```python
from build123d import *

# Parameters (mm, degrees)
SKETCH_1_R          = 15
EXTRUDE_1_DEPTH     = 6
SKETCH_2_R          = 1.6
CUT_EXTRUDE_1_DEPTH = 23.045407685
SKETCH_3_R          = 3.05
CUT_EXTRUDE_2_DEPTH = 1.2
SKETCH_4_R          = 4
EXTRUDE_2_DEPTH     = 25


with BuildPart() as part:
    # 草图1 → 凸台-拉伸1 (new body)
    with BuildSketch(Plane.XY):
        Circle(SKETCH_1_R)
    extrude(amount=EXTRUDE_1_DEPTH)

    # 草图2 → 切除-拉伸1 (cut, through all)
    with BuildSketch(Plane.XY.offset(6)):
        with Locations((0, 11.5)):
            Circle(SKETCH_2_R)
        with Locations((9.959292144, -5.75)):
            Circle(SKETCH_2_R)
        with Locations((-9.959292144, -5.75)):
            Circle(SKETCH_2_R)
        with Locations((-9.09326674, 5.25)):
            Circle(SKETCH_2_R)
        with Locations((9.09326674, 5.25)):
            Circle(SKETCH_2_R)
        with Locations((0, -10.5)):
            Circle(SKETCH_2_R)
    extrude(amount=-CUT_EXTRUDE_1_DEPTH, mode=Mode.SUBTRACT)

    # 草图3 → 切除-拉伸2 (cut)
    with BuildSketch(Plane.XY.offset(6)):
        with Locations((-9.09326674, 5.25)):
            Circle(SKETCH_3_R)
        with Locations((0, 11.5)):
            Circle(SKETCH_3_R)
        with Locations((9.09326674, 5.25)):
            Circle(SKETCH_3_R)
        with Locations((9.959292144, -5.75)):
            Circle(SKETCH_3_R)
        with Locations((0, -10.5)):
            Circle(SKETCH_3_R)
        with Locations((-9.959292144, -5.75)):
            Circle(SKETCH_3_R)
    extrude(amount=-CUT_EXTRUDE_2_DEPTH, mode=Mode.SUBTRACT)

    # 草图4 → 凸台-拉伸2 (add)
    with BuildSketch(Plane.XY.offset(6)):
        Circle(SKETCH_4_R)
    extrude(amount=EXTRUDE_2_DEPTH)

    # 草图5 → 旋转2 (revolve)
    with BuildSketch(Plane(origin=(0, 0, 0), x_dir=(1, 0, 0), z_dir=(0, 1, 0))):
        with BuildLine():
            Line((0, -29), (0, -45.9))
            ThreePointArc((0, -45.9), (-8.45, -37.45), (0, -29))
        make_face()
    revolve(axis=Axis((0, 0, 0), (0, 0, 1)))


solid = part.part
```
Input: part model. Units: mm. Frame: model coordinates. A direction names the side the tool comes from. Give positions to 0.01 mm unless a question says otherwise; leave off trailing zeros. Order: outer loops, then holes, each group sorted by start corner. A loop starts at its lowest first (then second) coordinate and runs counter-clockwise, first axis right, second up.
1. Material intervals for L1, parallel to Y at x = 0, z = 1.2; L2, parallel to Y at x = 0, z = 5.75; L3, parallel to Z at x = -5.75, y = 12.75, sorted ascending.
Derived:
L1: y = -15 to -12.1, -8.9 to 9.9, 13.1 to 15
L2: y = -15 to -13.55, -7.45 to 8.45, 14.55 to 15
L3: z = 0 to 6
2. Section B-B on y = 0. Return the cut outline in (x, z), and give its area (3 significant figures).
Derived:
outline: (-15, 0) - (15, 0) - (15, 6) - (4, 6) - (4, 30.01) arc R8.45 ccw (long way) to (-4, 30.01) - (-4, 6) - (-15, 6) - close
area: 591 mm2
3. Reachability of faces 5 (the cylindrical face through (-10.69, 5.32, 2.43)), 6 (the cylindrical face through (12.777, -6.918, 5.408)), 7 (the cylindrical face through (8.432, 2.273, 5.408)) from +Z, -Z, +X, -X, +Y, -Y: full face, straight path, thin tool, end or side. Return the list, or none.
Derived:
face 5: +Z, -Z
face 6: +Z
face 7: none
4. Section D-D on y = 5.25. Return the cut outline in (x, z), and give its area (3 significant figures).
Derived:
outline: (-14.05, 0) - (-10.69, 0) - (-10.69, 4.8) - (-12.14, 4.8) - (-12.14, 6) - (-14.05, 6) - close; (-7.49, 0) - (7.49, 0) - (7.49, 4.8) - (6.04, 4.8) - (6.04, 6) - (-6.04, 6) - (-6.04, 4.8) - (-7.49, 4.8) - close; circle Ø13.24 at (0, 37.45); (10.69, 0) - (14.05, 0) - (14.05, 6) - (12.14, 6) - (12.14, 4.8) - (10.69, 4.8) - close
area: 261 mm2
5. Section A-A on x = 0. Return the cut outline in (y, z).
Derived:
outline: (-15, 0) - (-12.1, 0) - (-12.1, 4.8) - (-13.55, 4.8) - (-13.55, 6) - (-15, 6) - close; (-8.9, 0) - (9.9, 0) - (9.9, 4.8) - (8.45, 4.8) - (8.45, 6) - (4, 6) - (4, 30.01) arc R8.45 ccw (long way) to (-4, 30.01) - (-4, 6) - (-7.45, 6) - (-7.45, 4.8) - (-8.9, 4.8) - close; (13.1, 0) - (15, 0) - (15, 6) - (14.55, 6) - (14.55, 4.8) - (13.1, 4.8) - close
6. Section C-C on z = 3. Return the cut outline in (x, y).
Derived:
outline: circle Ø30 at (0, 0); hole circle Ø3.2 at (-9.96, -5.75); hole circle Ø3.2 at (-9.09, 5.25); hole circle Ø3.2 at (0, -10.5); hole circle Ø3.2 at (0, 11.5); hole circle Ø3.2 at (9.09, 5.25); hole circle Ø3.2 at (9.96, -5.75)
7. Mould query, pull axis X, two halves, no side actions, for faces 1 (the cylindrical face through (-12.38, -7.606, 5.408)), 2 (the flat face through (0, 0, 0)), 3 (the cylindrical face through (-8.48, -6.36, 2.43)), 4 (the cylindrical face through (-0.867, -3.905, 17.835)). Classes: released by +X, released by -X, zero draft, split by the parting line, or undercut.
Derived:
face 1: undercut
face 2: zero draft
face 3: undercut
face 4: split by the parting line
8. Pin query (flat end, axial travel): pin 1 (3.5 mm diameter, centred on x = 0, y = 11.5, fed in from +Z); pin 2 (8 mm diameter, centred on x = 0, y = -10.5, fed in from +Z); pin 3 (3 mm diameter, centred on x = -0.5, y = 10, fed in from +Z); pin 4 (10 mm diameter, centred on x = 9.09, y = 5.25, fed in from -Z). Return the tip coordinate at first contact, or that it passes through.
Derived:
pin 1: stops at z = 4.8
pin 2: stops at z = 42.85
pin 3: stops at z = 6
pin 4: stops at z = 0
